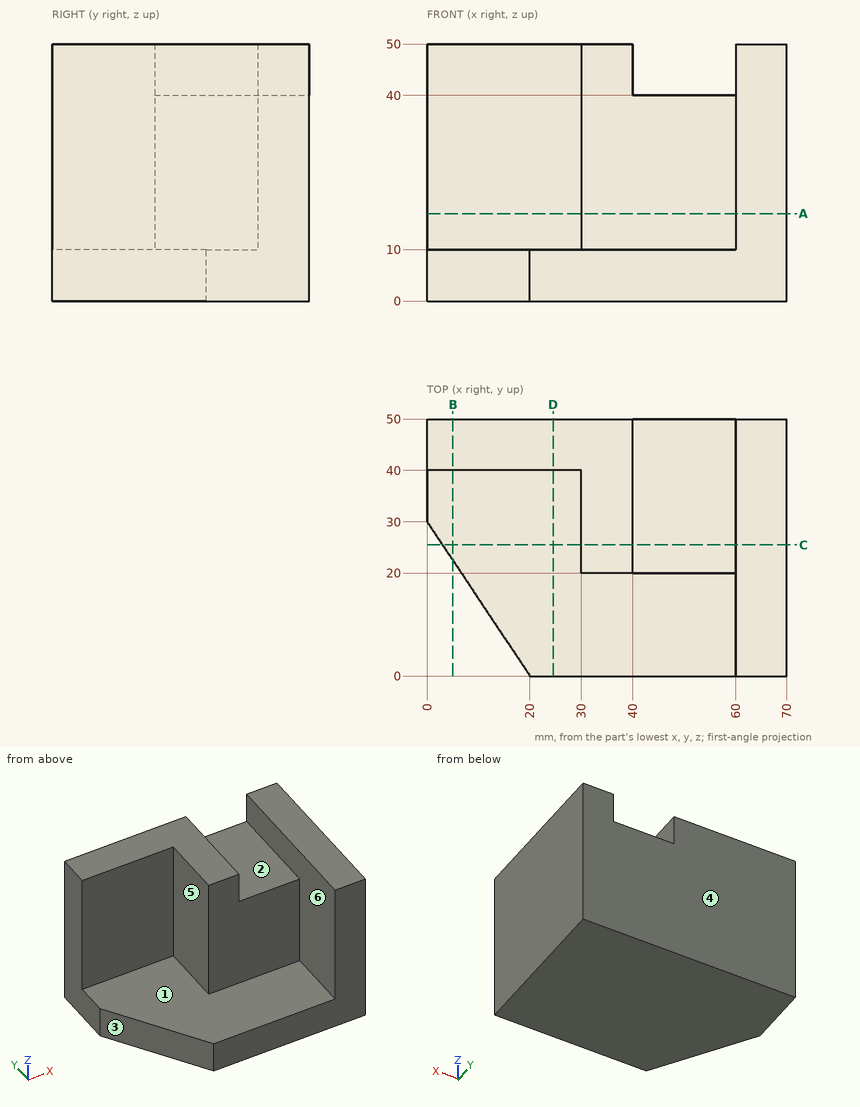
Design review of the part shown in the three views and the two pictorial views. Dimensions are in mm from the part's minimum x, y and z. A direction names the side the tool comes from. Round coordinates to 2 decimals unless told otherwise and drop trailing zeros. Loops run counter-clockwise (first coordinate to the right, second up) from the corner with the lowest first, then second, coordinate; pieces in that order, holes last. Notation, with made-up numbers: (28, 6) -> (35, 6) arc R26 cw to (35, 41) -> close; hole circle Ø6 at (53.25, -19.5). An arc over 180 degrees is marked (long way). Answer as CSV lines item,"result".
1) Draft analysis for pull direction X (two halves, no side actions). For the marked faces 1, 2 and 3, state which applies: pulls with the +X half, pulls with the -X half, needs draft (parallel to the pull), parting line crosses it, or undercut.
Geometry results:
face 1,"needs draft"
face 2,"undercut"
face 3,"pulls with the -X half"
2) To check wall thickness, follow line 1 along X through (y, z) = (48, 42); line 2 along X through (y, z) = (35, 40.5); line 3 along X through (y, z) = (18.5, 14). State the ranges of each line that lie inside material, in increasing order. Write a range as from..to.
Geometry results:
line 1,"x = 0..40, 60..70"
line 2,"x = 30..40, 60..70"
line 3,"x = 60..70"
3) For P1, Ø4, axis at x = 19, y = 37.5, coming from the +Z side; P2, Ø15, axis at x = 22, z = 35, coming from the -Y side; P3, Ø6, axis at x = 50, y = 40.5, coming from the +Z side, all flat-tipped, find the tip position at first contact; note any pin that passes through.
Geometry results:
P1,"stops at z = 10"
P2,"stops at y = 40"
P3,"stops at z = 40"
4) Tool access review of the marked faces 4, 5 and 6: name each direction out of +Z, -Z, +X, -X, +Y, -Y from which nothing blocks a thin tool from reaching the whole face with its end or side.
Geometry results:
face 4,"+Z, -Z, +X, -X, +Y"
face 5,"+Z, -X, -Y"
face 6,"+Z, -Y"
5) Add section B-B on x = 5. Write out the cut boundary in (y, z).
Geometry results:
outline,"(22.5, 0) -> (50, 0) -> (50, 50) -> (40, 50) -> (40, 10) -> (22.5, 10) -> close"
6) Add section C-C on y = 25.5. Write out the cut boundary in (x, z).
Geometry results:
outline,"(3, 0) -> (70, 0) -> (70, 50) -> (60, 50) -> (60, 40) -> (40, 40) -> (40, 50) -> (30, 50) -> (30, 10) -> (3, 10) -> close"
7) Add section D-D on x = 24.5. Write out the cut boundary in (y, z), plus the area to 3 significant figures.
Geometry results:
outline,"(0, 0) -> (50, 0) -> (50, 50) -> (40, 50) -> (40, 10) -> (0, 10) -> close"
area,"900 mm²"
8) Add section A-A on z = 17. Write out the cut boundary in (x, y), plus the area to 3 significant figures.
Geometry results:
outline,"(0, 40) -> (30, 40) -> (30, 20) -> (60, 20) -> (60, 0) -> (70, 0) -> (70, 50) -> (0, 50) -> close"
area,"1,700 mm²"
